Geometry: see drawing. Coordinates: mm, zero at the bounding-box minimum. Give positions to 0.01 mm unless a question says otherwise; leave off trailing zeros. Write each loop counter-clockwise with the first axis right and the second up, starting at its lowest first coordinate (ties: lowest second). Pieces come first, ordered by that corner, then holes. Notation, with made-up numbers: (0, -10.75) -> (55, -10.75) arc R23 cw to (55, 4.25) -> close; hole circle Ø1 at (61.5, 68). An arc over 180 degrees is marked (long way). Answer as a JSON object with one key per item and string values. Group by question number.
Item 1: Section query D-D on z = 180.5. Return the cut outline in (x, y).
Item 2: Ray query, probe 1 along X at (y, z) = (3.75, 101.5); probe 2 along X at (y, z) = (3.25, 159.5); probe 3 along Z at (x, y) = (961.5, 1). Return the intervals inside material, ascending. Write a range as from..to.
Item 3: Section query B-B on y = 3.75. Return the cut outline in (x, z).
Item 4: First-contact query: pin 1 Ø5 at (x, y) = (13, 4) entering from +Z; pin 2 Ø3 at (y, z) = (6.5, 17.5) entering from -X; pin 3 Ø3 at (y, z) = (6, 179) entering from +X. Flat tips, straight axial feed; report the tip coordinate or a pass-through.
Item 5: Section query A-A on z = 72. Return the cut outline in (x, y).
Item 6: Section query C-C on z = 16.5. Return the cut outline in (x, y).
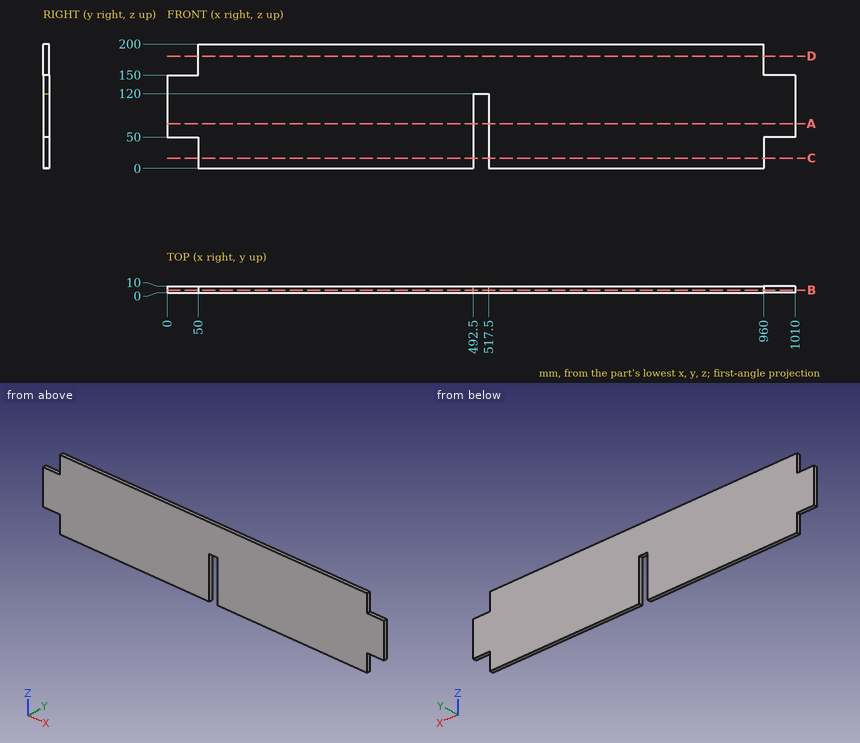
Worked answers:
{
 "1": {"outline": "(50, 0) -> (960, 0) -> (960, 10) -> (50, 10) -> close"},
 "2": {"probe 1": "0..492.5, 517.5..1010", "probe 2": "50..960", "probe 3": "50..150"},
 "3": {"outline": "(0, 50) -> (50, 50) -> (50, 0) -> (492.5, 0) -> (492.5, 120) -> (517.5, 120) -> (517.5, 0) -> (960, 0) -> (960, 50) -> (1010, 50) -> (1010, 150) -> (960, 150) -> (960, 200) -> (50, 200) -> (50, 150) -> (0, 150) -> close"},
 "4": {"pin 1": "z = 150", "pin 2": "x = 50", "pin 3": "x = 960"},
 "5": {"outline": "(0, 0) -> (492.5, 0) -> (492.5, 10) -> (0, 10) -> close; (517.5, 0) -> (1010, 0) -> (1010, 10) -> (517.5, 10) -> close"},
 "6": {"outline": "(50, 0) -> (492.5, 0) -> (492.5, 10) -> (50, 10) -> close; (517.5, 0) -> (960, 0) -> (960, 10) -> (517.5, 10) -> close"}
}
